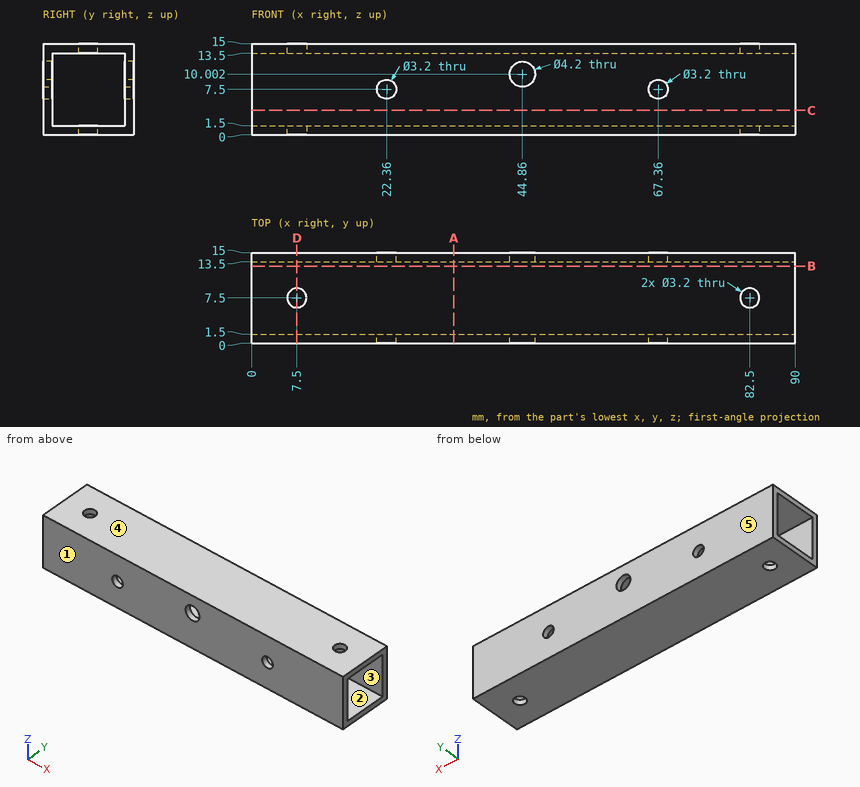
The drawing under review shows one solid part. Ordinate dimensions are in mm from its lowest x, y, z. A direction names the side the tool comes from. Give positions to 0.01 mm unless a question says otherwise; leave off trailing zeros. Write each loop counter-clockwise with the first axis right and the second up, starting at its lowest first coordinate (ties: lowest second). Pieces come first, ordered by that corner, then holes. Notation, with made-up numbers: (-8, 17.25) -> (21, 17.25) arc R13 ccw to (21, 35.25) -> close; hole circle Ø10 at (55.5, 69.5). An arc over 180 degrees is marked (long way). Use CSV: the item, a comma, the result in double quotes.
Q1. Tool access review of the marked faces 1 and 2: name each direction out of +Z, -Z, +X, -X, +Y, -Y from which nothing blocks a thin tool from reaching the whole face with its end or side.
Conclusion:
face 1,"+Z, -Z, +X, -X, -Y"
face 2,"+X, -X"
Q2. To check wall thickness, follow probe 1 along X at (y, z) = (14.1, 7.5); probe 2 along Z at (x, y) = (59, 12.25). State the ranges of each line that lie inside material, in increasing order. Write a range as [from, to].
Conclusion:
probe 1,"[0, 20.76], [23.96, 65.76], [68.96, 90]"
probe 2,"[0, 1.5], [13.5, 15]"
Q3. Mouldability with a two-part tool opening along Y and no side actions: class the marked faces 3, 4 and 5 as pulls with the +Y half, pulls with the -Y half, needs draft (parallel to the pull), parting line crosses it, or undercut.
Conclusion:
face 3,"undercut"
face 4,"needs draft"
face 5,"pulls with the +Y half"
Q4. Take a section at B-B, the plane y = 12.75. Write out the cut boundary in (x, z).
Conclusion:
outline,"(0, 0) -> (90, 0) -> (90, 1.5) -> (0, 1.5) -> close; (0, 13.5) -> (90, 13.5) -> (90, 15) -> (0, 15) -> close"
Q5. Take a section at A-A, the plane x = 33.5. Write out the cut boundary in (y, z).
Conclusion:
outline,"(0, 0) -> (15, 0) -> (15, 15) -> (0, 15) -> close; hole (1.5, 1.5) -> (13.5, 1.5) -> (13.5, 13.5) -> (1.5, 13.5) -> close"
Q6. Take a section at D-D, the plane x = 7.5. Write out the cut boundary in (y, z).
Conclusion:
outline,"(0, 0) -> (5.9, 0) -> (5.9, 1.5) -> (1.5, 1.5) -> (1.5, 13.5) -> (5.9, 13.5) -> (5.9, 15) -> (0, 15) -> close; (9.1, 0) -> (15, 0) -> (15, 15) -> (9.1, 15) -> (9.1, 13.5) -> (13.5, 13.5) -> (13.5, 1.5) -> (9.1, 1.5) -> close"
Q7. For P1, Ø1.9, axis at x = 22.36, z = 7.5, coming from the -Y side, flat-tipped, find the tip position at first contact; note if it passes through.
Conclusion:
P1,"through"
